Work out the finished part from the listing and answer in its coordinate system (mm). A direction names the side the tool comes from. Coordinates: 2 decimals unless noted, no trailing zeros. Order: outer loops, then holes, each group sorted by start corner. A loop starts at its lowest first (then second) coordinate and runs counter-clockwise, first axis right, second up. Notation, with made-up numbers: M 80.5,47.5 L 96.5,47.5 A6 ccw 96.5,53.5 Z; hole C -25.5,80 d9. An arc over 180 degrees is marked long. Use a Markdown table: item, result.
from build123d import *

# Parameters (mm, degrees)
F0_R     = 2.15
F0_R_2   = 4
F1_DEPTH = 10
F0_R_3   = 4.5
F0_R_4   = 4.55
F2_DEPTH = 20
F3_START = 17
F0_R_5   = 1.55
F3_DEPTH = 3
F4_R     = 6
F5_R     = 3


with BuildPart() as f1:
    # F0 (on Top) → F1 (new body)
    with BuildSketch(Plane.XY):
        Polygon((73.3899642625, 49.4741697694), (-13.6100357375, 49.4741697694), (-13.6100357375, 2.4741697694), (73.3899642625, 2.4741697694), (73.3899642625, 36.8359796703), align=None)
        with Locations((-7.6100357375, 8.4741697694)):
            Circle(F0_R, mode=Mode.SUBTRACT)
        Polygon((-0.0100357375, 4.4741697694), (-0.0100357375, 47.4741697694), (30.4899642625, 47.4741697694), (30.4899642625, 4.4741697694), (20.6151821792, 4.4741697694), (8.9151821792, 4.4741697694), align=None, mode=Mode.SUBTRACT)
        with Locations((67.3899642625, 8.4741697694)):
            Circle(F0_R, mode=Mode.SUBTRACT)
        with Locations((-7.6100357375, 43.4741697694)):
            Circle(F0_R, mode=Mode.SUBTRACT)
        Polygon((30.8899642625, 4.4741697694), (30.8899642625, 47.4741697694), (61.3899642625, 47.4741697694), (61.3899642625, 4.4741697694), (53.5151823588, 4.4741697694), (41.8151823588, 4.4741697694), align=None, mode=Mode.SUBTRACT)
        with Locations((67.3899642625, 43.4741697694)):
            Circle(F0_R, mode=Mode.SUBTRACT)
        with BuildLine():
            add(Edge.make_bspline(
                [(73.3899642625, 2.4741697694), (104.1805148125, 2.9646980111), (103.3740565181, 22.3197154701), (73.3899642625, 36.8359796703)],
                knots=[0, 0, 0, 0, 34.3618099009, 34.3618099009, 34.3618099009, 34.3618099009], degree=3))
            Line((73.3899642625, 36.8359796703), (73.3899642625, 2.4741697694))
        make_face()
        with Locations((85.3899642625, 14.960267581)):
            Circle(F0_R_2, mode=Mode.SUBTRACT)
    extrude(amount=F1_DEPTH)

    # F0 (on Top) → F2 (join)
    with BuildSketch(Plane.XY):
        Polygon((30.4899642625, 47.4741697694), (-0.0100357375, 47.4741697694), (-0.0100357375, 4.4741697694), (8.9151821792, 4.4741697694), (20.6151821792, 4.4741697694), (30.4899642625, 4.4741697694), align=None)
        with Locations((24.2899642625, 10.4741697694)):
            Circle(F0_R_3, mode=Mode.SUBTRACT)
        with Locations((8.7899642625, 25.9741697694)):
            Circle(F0_R_4, mode=Mode.SUBTRACT)
        with Locations((24.2899642625, 41.4741697694)):
            Circle(F0_R_3, mode=Mode.SUBTRACT)
        Polygon((61.3899642625, 47.4741697694), (30.8899642625, 47.4741697694), (30.8899642625, 4.4741697694), (41.8151823588, 4.4741697694), (53.5151823588, 4.4741697694), (61.3899642625, 4.4741697694), align=None)
        with Locations((39.6899642625, 25.9741697694)):
            Circle(F0_R_4, mode=Mode.SUBTRACT)
        with Locations((55.1899642625, 10.4741697694)):
            Circle(F0_R_3, mode=Mode.SUBTRACT)
        with Locations((55.1899642625, 41.4741697694)):
            Circle(F0_R_3, mode=Mode.SUBTRACT)
    extrude(amount=F2_DEPTH)

    # F0 (on Top) → F3 (join)
    with BuildSketch(Plane.XY.offset(F3_START)):
        with Locations((24.2899642625, 41.4741697694)):
            Circle(F0_R_3)
        with Locations((24.2899642625, 41.4741697694)):
            Circle(F0_R_5, mode=Mode.SUBTRACT)
        with Locations((55.1899642625, 41.4741697694)):
            Circle(F0_R_3)
        with Locations((55.1899642625, 41.4741697694)):
            Circle(F0_R_5, mode=Mode.SUBTRACT)
        with Locations((55.1899642625, 10.4741697694)):
            Circle(F0_R_3)
        with Locations((55.1899642625, 10.4741697694)):
            Circle(F0_R_5, mode=Mode.SUBTRACT)
        with Locations((24.2899642625, 10.4741697694)):
            Circle(F0_R_3)
        with Locations((24.2899642625, 10.4741697694)):
            Circle(F0_R_5, mode=Mode.SUBTRACT)
    extrude(amount=F3_DEPTH)

    # F4
    f4_edges = [f1.edges().sort_by_distance(p)[0] for p in [
        (73.389964, 2.47417, 5),
        (73.389964, 49.47417, 5),
        (-13.610036, 49.47417, 5),
        (-13.610036, 2.47417, 5),
    ]]
    fillet(f4_edges, radius=F4_R)

    # F5
    f5_edges = [f1.edges().sort_by_distance(p)[0] for p in [
        (-0.010036, 4.47417, 15),
        (61.389964, 4.47417, 15),
        (61.389964, 47.47417, 15),
        (-0.010036, 47.47417, 15),
    ]]
    fillet(f5_edges, radius=F5_R)


solid = f1.part
1. Find the intervals of material crossed by probe 1 along X at (y, z) = (17.5, 18.75); probe 2 along X at (y, z) = (14.5, 2.5); probe 3 along X at (y, z) = (9.5, 14.5), in increasing order.
Answers below:
| item | result |
|---|---|
| probe 1 | -0.01 to 30.49, 30.89 to 61.39 |
| probe 2 | -13.61 to 22.28, 26.3 to 53.18, 57.2 to 81.42, 89.36 to 96.18 |
| probe 3 | -0.01 to 19.9, 28.68 to 30.49, 30.89 to 50.8, 59.58 to 61.39 |
2. Section B-B on y = 38 is taken. Determine the outline of the cut face in (x, z), then the cut area to 3 significant figures.
Answers below:
| item | result |
|---|---|
| outline | M -13.61,0 L 21.43,0 L 21.43,17 L 27.15,17 L 27.15,0 L 52.33,0 L 52.33,17 L 58.05,17 L 58.05,0 L 73.39,0 L 73.39,10 L 61.39,10 L 61.39,20 L 30.89,20 L 30.89,10 L 30.49,10 L 30.49,20 L -0.01,20 L -0.01,10 L -13.61,10 Z |
| area | 1,290 mm² |
3. Section A-A on x = 36.5 is taken. Determine the outline of the cut face in (y, z).
Answers below:
| item | result |
|---|---|
| outline | M 2.47,0 L 22.73,0 L 22.73,20 L 4.47,20 L 4.47,10 L 2.47,10 Z; M 29.22,0 L 49.47,0 L 49.47,10 L 47.47,10 L 47.47,20 L 29.22,20 Z |
4. For a pull along Y with two mould halves and no side action, classify faces 1 (the face through (44, 4.474, 15)), 2 (the face through (23.704, 45.936, 8.381)), 3 (the face through (15, 26, 20)) as +Y half, -Y half, draft (parallel to the pull), parting line (faces both ways), or undercut.
Answers below:
| item | result |
|---|---|
| face 1 | -Y half |
| face 2 | undercut |
| face 3 | draft |
5. For faces 4 (the face through (61.39, 26, 15)), 5 (the face through (17, 47.474, 15)), 6 (the face through (73.39, 40, 5)), 7 (the face through (24.2, 39.5, 17)), determine the directions among +Z, -Z, +X, -X, +Y, -Y from which every point of the face is accessible in a straight line to the end or side of a thin tool.
Answers below:
| item | result |
|---|---|
| face 4 | +Z, +X, +Y, -Y |
| face 5 | +Z, +X, -X, +Y |
| face 6 | +Z, -Z, +X, +Y |
| face 7 | -Z |
6. Flat-ended cylindrical pins translate along their axes: P1, Ø5, axis at x = 46, z = 16.5, coming from the +Y side; P2, Ø3, axis at x = 47, z = 14.5, coming from the -Y side; P3, Ø3, axis at x = 24.29, y = 10.47, coming from the -Z side; P4, Ø10, axis at y = 21.5, z = 9.5, coming from the +X side. Find the tip coordinate at first contact, or state that the pin passes through.
Answers below:
| item | result |
|---|---|
| P1 | y = 47.47 |
| P2 | y = 4.47 |
| P3 | through |
| P4 | x = 95.91 |
7. Section C-C on y = 23.5 is taken. Give the number of separate pieces and of enclosed holes in the cut face, then the cut area to 3 significant figures.
Answers below:
| item | result |
|---|---|
| separate pieces | 3 |
| enclosed holes | 0 |
| area | 1,360 mm² |
